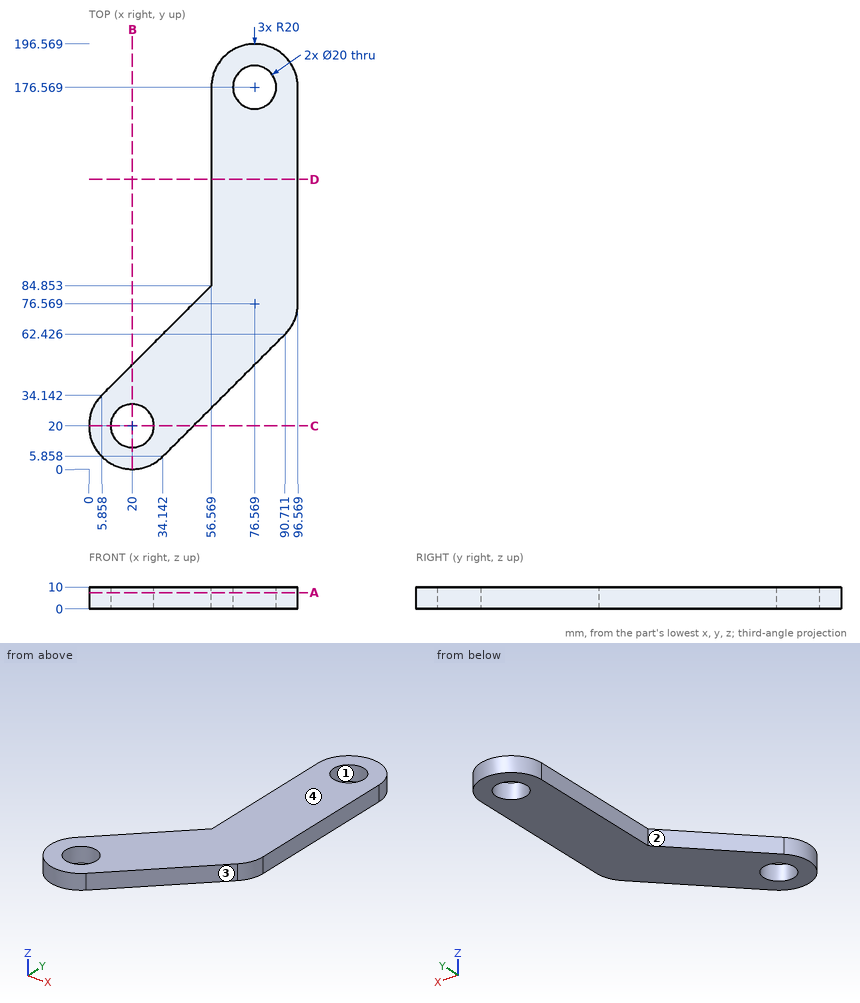
Study the drawing (mm; zero at the part's minimum x, y, z) and answer. Give positions to 0.01 mm unless a question says otherwise; leave off trailing zeros. Order: outer loops, then holes, each group sorted by start corner. A loop starts at its lowest first (then second) coordinate and runs counter-clockwise, first axis right, second up.
1) Find section A-A on z = 7.5. Write down the section's boundary in (x, y).
Reported:
outline: (5.86, 34.14) arc R20 ccw to (34.14, 5.86) - (90.71, 62.43) arc R20 ccw to (96.57, 76.57) - (96.57, 176.57) arc R20 ccw to (56.57, 176.57) - (56.57, 84.85) - close; hole circle Ø20 at (20, 20); hole circle Ø20 at (76.57, 176.57)
2) Determine the mould class of the marked faces 1, 2, 3 and 4 for opening direction Y: pulls with the +Y half, pulls with the -Y half, needs draft (parallel to the pull), parting line crosses it, or undercut.
Reported:
face 1: undercut
face 2: pulls with the +Y half
face 3: pulls with the -Y half
face 4: needs draft
3) Find section D-D on y = 134. Write down the section's boundary in (x, z).
Reported:
outline: (56.57, 0) - (96.57, 0) - (96.57, 10) - (56.57, 10) - close
4) Consider line 1 along Y through (x, z) = (20, 3.75) (1 decimal); line 2 along Y through (x, z) = (82.5, 5.25) (1 decimal); line 3 along X through (y, z) = (131, 7). Determine where each line is inside the solid, lowest interval first.
Reported:
line 1: y = 0 to 10, 30 to 48.3
line 2: y = 54.2 to 168.5, 184.6 to 195.7
line 3: x = 56.57 to 96.57
5) Find section B-B on x = 20. Write down the section's boundary in (y, z) (1 decimal), then the cut area to 3 significant figures.
Reported:
outline: (0, 0) - (10, 0) - (10, 10) - (0, 10) - close; (30, 0) - (48.3, 0) - (48.3, 10) - (30, 10) - close
area: 283 mm2
6) Given P1, Ø3, axis at x = 63, z = 3, coming from the -Y side (1 decimal); P2, Ø2, axis at y = 50, z = 1, coming from the -X side (1 decimal); P3, Ø2, axis at x = 47, z = 2.5, coming from the -Y side (1 decimal); P4, Ø12, axis at x = 20, y = 20, coming from the -Z side, each flat-ended and moving along its own axis, determine where each tip first touches the part or whether it passes through.
Reported:
P1: stops at y = 33.2
P2: stops at x = 20.7
P3: stops at y = 17.7
P4: passes through
